Build history of the part. All positions in model axes, mm. A direction names the side the tool comes from. Give positions to 0.01 mm unless a question says otherwise; leave off trailing zeros. Order: outer loops, then holes, each group sorted by start corner. A loop starts at its lowest first (then second) coordinate and runs counter-clockwise, first axis right, second up. Notation, with made-up numbers: (21, 19.25) -> (51, 19.25) arc R14 ccw to (51, 43.25) -> close; hole circle Ø8 at (23, 17.25). An arc over 180 degrees is marked (long way). Use a Markdown table: item, result. Add a question column.
```python
from build123d import *

# Parameters (mm, degrees)
EXTRUDE_1_DEPTH       = 3.3
SKETCH_1_3_W          = 29.5
SKETCH_1_3_H          = 13
EXTRUDE_2_DEPTH       = 21.6
SKETCH_3_W            = 29.5
SKETCH_3_H            = 13
CUT_EXTRUDE_1_DEPTH   = 14.4
SKETCH_4_W            = 7.25988549
SKETCH_4_H            = 9.71067486
CUT_EXTRUDE_2_DEPTH   = 4.4
SKETCH_5_W            = 10.1
SKETCH_5_H            = 1.2
EXTRUDE_3_DEPTH       = 8.2
EXTRUDE_4_OUTLINE_W   = 6.05761146
EXTRUDE_4_OUTLINE_H   = 3.941693248
EXTRUDE_4_OUTLINE_W_2 = 5.05761146
EXTRUDE_4_OUTLINE_H_2 = 2.2
EXTRUDE_4_DEPTH       = 7.5
SKETCH_6_R            = 1.6
CUT_EXTRUDE_3_DEPTH   = 7.5


# Read off the part's stored shape, not the designer's step: 凸台-拉伸4
with BuildPart() as part:
    # 草图1 → 凸台-拉伸1 (new body)
    with BuildSketch(Plane.XY):
        with BuildLine():
            ThreePointArc((-18.5, 3.75), (-22.25, 0), (-18.5, -3.75))
            Line((-18.5, -3.75), (-18.5, 3.75))
        make_face()
        with BuildLine():
            Line((-18.5, 3.75), (-18.5, -3.75))
            ThreePointArc((-18.5, -3.75), (-15.848349571, -2.651650429), (-14.75, 0))
            ThreePointArc((-14.75, 0), (-15.848349571, 2.651650429), (-18.5, 3.75))
        make_face()
        with BuildLine():
            Line((-14.75, 3.75), (-18.5, 3.75))
            ThreePointArc((-18.5, 3.75), (-15.848349571, 2.651650429), (-14.75, 0))
            Line((-14.75, 0), (-14.75, 3.75))
        make_face()
        with BuildLine():
            ThreePointArc((-14.75, 0), (-15.848349571, -2.651650429), (-18.5, -3.75))
            Line((-18.5, -3.75), (-14.75, -3.75))
            Line((-14.75, -3.75), (-14.75, 0))
        make_face()
        Polygon((-14.75, 0), (-14.75, -3.75), (14.75, -3.75), (14.75, -4e-09), (14.75, 3.75), (-14.75, 3.75), align=None)
        with BuildLine():
            ThreePointArc((14.75, -4e-09), (15.848349572, -2.651650431), (18.5, -3.75))
            Line((18.5, -3.75), (18.5, 3.75))
            ThreePointArc((18.5, 3.75), (15.848349569, 2.651650428), (14.75, -4e-09))
        make_face()
        with BuildLine():
            Line((18.5, 3.75), (18.5, -3.75))
            ThreePointArc((18.5, -3.75), (21.151650429, -2.651650429), (22.25, 0))
            ThreePointArc((22.25, 0), (21.151650429, 2.651650429), (18.5, 3.75))
        make_face()
        with BuildLine():
            Line((14.75, 3.75), (14.75, -4e-09))
            ThreePointArc((14.75, -4e-09), (15.848349569, 2.651650428), (18.5, 3.75))
            Line((18.5, 3.75), (14.75, 3.75))
        make_face()
        with BuildLine():
            Line((14.75, -4e-09), (14.75, -3.75))
            Line((14.75, -3.75), (18.5, -3.75))
            ThreePointArc((18.5, -3.75), (15.848349572, -2.651650431), (14.75, -4e-09))
        make_face()
    extrude(amount=EXTRUDE_1_DEPTH)

    # 草图1<3> → 凸台-拉伸2 (add)
    with BuildSketch(Plane.XY):
        Rectangle(SKETCH_1_3_W, SKETCH_1_3_H)
    extrude(amount=EXTRUDE_2_DEPTH)

    # 草图3 → 切除-拉伸1 (cut)
    with BuildSketch(Plane.XY.offset(21.6)):
        Rectangle(SKETCH_3_W, SKETCH_3_H)
        Polygon((-14.375, -5.95), (-14.375, 5.95), (-5.425, 5.95), (-5.425, 4.2), (5.425, 4.2), (5.425, 5.95), (14.375, 5.95), (14.375, -5.95), (5.425, -5.95), (5.425, -4.2), (-5.425, -4.2), (-5.425, -5.95), align=None, mode=Mode.SUBTRACT)
    extrude(amount=-CUT_EXTRUDE_1_DEPTH, mode=Mode.SUBTRACT)

    # 草图4 → 切除-拉伸2 (cut)
    with BuildSketch(Plane.XY.offset(21.6)):
        with Locations((-9.941881404, -0.092482618)):
            Rectangle(SKETCH_4_W, SKETCH_4_H)
        with Locations((9.941881404, -0.092482618)):
            Rectangle(SKETCH_4_W, SKETCH_4_H)
    extrude(amount=-CUT_EXTRUDE_2_DEPTH, mode=Mode.SUBTRACT)

    # 草图5 → 凸台-拉伸3 (add)
    with BuildSketch(Plane.XZ.offset(4.2)):
        with Locations((0, 3.9)):
            Rectangle(SKETCH_5_W, SKETCH_5_H)
    extrude(amount=EXTRUDE_3_DEPTH)

    # 凸台-拉伸4 outline → 凸台-拉伸4 (add)
    with BuildSketch(Plane.XZ.offset(4.2)):
        with Locations((0, 6.470846624)):
            Rectangle(EXTRUDE_4_OUTLINE_W, EXTRUDE_4_OUTLINE_H)
        with Locations((0, 6.1)):
            Rectangle(EXTRUDE_4_OUTLINE_W_2, EXTRUDE_4_OUTLINE_H_2, mode=Mode.SUBTRACT)
    extrude(amount=EXTRUDE_4_DEPTH)

    # 草图6 → 切除-拉伸3 (cut)
    with BuildSketch(Plane.XY.offset(3.3)):
        with Locations((-18.5, 0)):
            Circle(SKETCH_6_R)
        with Locations((18.5, 0)):
            Circle(SKETCH_6_R)
    extrude(amount=-CUT_EXTRUDE_3_DEPTH, mode=Mode.SUBTRACT)


solid = part.part
```
(1) Band-saw the part on A-A on z = 17.75. Give the cut face in (x, y) (3 decimals).
(2) Pin check, flat tips, straight feed: pin 1 Ø5 at (y, z) = (-2.5, 10) entering from -X (3 decimals); pin 2 Ø3 at (x, z) = (-13.5, 13) entering from +Y; pin 3 Ø2.5 at (x, z) = (8, 12.5) entering from -Y. Stop position of each tip, or through.
(3) Band-saw the part on B-B on y = 5.25. Give the cut face in (x, z) (3 decimals), plus the area to 3 significant figures.
(4) Mould opens along X. For faces 5 (the face through (-5.425, 5, 15)), 6 (the face through (-14.375, 0, 15)), 7 (the face through (0, 0, 21.6)) say: released by +X, released by -X, zero draft, split by the parting line, or undercut.
(5) Tool access for faces 1 (the face through (14.375, 0, 15)), 2 (the face through (-17, 3.75, 2)), 3 (the face through (-5.425, -5, 15)), 4 (the face through (5.05, -9, 4)): list every direction of +Z, -Z, +X, -X, +Y, -Y with a clear straight run to the whole face (end or side of a thin tool).
(6) Band-saw the part on C-C on x = 9. Give the cut face in (y, z), plus the area to 3 significant figures.
(7) Wall check: probe 1 along Y at (x, z) = (18.5, 0.7); probe 2 along X at (y, z) = (-5.25, 16.5) (3 decimals). Give the ranges that are in metal, low to high.
Response:
| question | item | result |
|---|---|---|
| 1 | outline | (-14.375, -5.95) -> (-5.425, -5.95) -> (-5.425, -4.2) -> (5.425, -4.2) -> (5.425, -5.95) -> (14.375, -5.95) -> (14.375, 5.95) -> (5.425, 5.95) -> (5.425, 4.2) -> (-5.425, 4.2) -> (-5.425, 5.95) -> (-14.375, 5.95) -> close; hole (-13.572, -4.948) -> (-6.312, -4.948) -> (-6.312, 4.763) -> (-13.572, 4.763) -> close; hole (6.312, -4.948) -> (13.572, -4.948) -> (13.572, 4.763) -> (6.312, 4.763) -> close |
| 2 | pin 1 | stops at x = -14.375 |
| 2 | pin 2 | stops at y = 5.95 |
| 2 | pin 3 | stops at y = -5.95 |
| 3 | outline | (-14.75, 0) -> (14.75, 0) -> (14.75, 7.2) -> (14.375, 7.2) -> (14.375, 21.6) -> (5.425, 21.6) -> (5.425, 7.2) -> (-5.425, 7.2) -> (-5.425, 21.6) -> (-14.375, 21.6) -> (-14.375, 7.2) -> (-14.75, 7.2) -> close |
| 3 | area | 470 mm² |
| 4 | face 5 | undercut |
| 4 | face 6 | released by -X |
| 4 | face 7 | zero draft |
| 5 | face 1 | +Z, +X, +Y, -Y |
| 5 | face 2 | +Z, -Z, -X, +Y |
| 5 | face 3 | +Z, -Y |
| 5 | face 4 | +Z, -Z, +X, -Y |
| 6 | outline | (-6.5, 0) -> (6.5, 0) -> (6.5, 7.2) -> (5.95, 7.2) -> (5.95, 21.6) -> (4.76, 21.6) -> (4.76, 17.2) -> (-4.95, 17.2) -> (-4.95, 21.6) -> (-5.95, 21.6) -> (-5.95, 7.2) -> (-6.5, 7.2) -> close |
| 6 | area | 222 mm² |
| 7 | probe 1 | y = -3.75 to -1.6, 1.6 to 3.75 |
| 7 | probe 2 | x = -14.375 to -5.425, 5.425 to 14.375 |
